Autodesk Inventor part; units mm, degrees
ref_plane "YZ Plane" through (0, 0, 0) normal (1, 0, 0) x (0, 1, 0)
ref_plane "XZ Plane" through (0, 0, 0) normal (0, 1, 0) x (-1, 0, 0)
ref_plane "XY Plane" through (0, 0, 0) normal (0, 0, 1) x (1, 0, 0)
sketch "Sketch1" plane through (0, 0, 0) normal (0, 1, 0) x (-1, 0, 0)
  line L0 (75, 0) -> (75, -100)
  line L1 (75, -100) -> (-75, -100)
  line L2 (-75, -100) -> (-75, 100)
  line L3 (-75, 100) -> (75, 100)
  line L4 (75, 100) -> (75, 0)
  line L5 (75, 100) -> (75, 70)
  line L6 (75, -100) -> (75, -70)
  line L7 (-75, -100) -> (-75, -70)
  line L8 (-75, 100) -> (-75, 70)
  line L9 (75, 70) -> (75, 50)
  line L10 (-75, 70) -> (-75, 50)
  line L11 (-75, -70) -> (-75, -50)
  line L12 (75, -70) -> (75, -50)
  line L13 (75, -70) -> (72.5, -70)
  line L14 (72.5, -70) -> (72.5, -50)
  line L15 (72.5, -50) -> (75, -50)
  line L16 (-75, -70) -> (-72.5, -70)
  line L17 (-72.5, -70) -> (-72.5, -50)
  line L18 (-72.5, -50) -> (-75, -50)
  line L19 (75, 70) -> (72.5, 70)
  line L20 (72.5, 70) -> (72.5, 50)
  line L21 (72.5, 50) -> (75, 50)
  line L22 (-75, 70) -> (-72.5, 70)
  line L23 (-72.5, 70) -> (-72.5, 50)
  line L24 (-72.5, 50) -> (-75, 50)
  line L25 (-75, -100) -> (-75, -97)
  line L26 (-75, -100) -> (-72, -100)
  circle A0 centre (-69.4679, -94.4422) radius 3
  circle A1 centre (69.3699, -94.4422) radius 3
  circle A2 centre (69.3699, 94.4217) radius 3
  circle A3 centre (-69.4679, 94.4217) radius 3
  line L27 (75, -50) -> (75, -35)
  line L28 (75, 50) -> (75, 35)
  line L29 (75, -35) -> (75, -25)
  line L30 (75, 35) -> (75, 25)
  line L31 (75, -25) -> (75, -21)
  line L32 (75, -21) -> (75, -17)
  line L33 (75, -17) -> (75, -13)
  line L34 (75, -13) -> (75, -9)
  line L35 (75, -9) -> (75, -5)
  line L36 (75, -5) -> (75, -1)
  line L37 (75, -1) -> (75, 3)
  line L38 (75, 3) -> (75, 7)
  line L39 (75, 7) -> (75, 11)
  line L40 (75, 11) -> (75, 15)
  line L41 (75, 15) -> (75, 19)
  line L42 (75, 19) -> (75, 23)
  circle A4 centre (60, 30) radius 5
  circle A5 centre (-60, 30) radius 5
  circle A6 centre (0, 30) radius 5
  line L43 (0, -35) -> (0, -30)
  circle A7 centre (0, -30) radius 5
  circle A8 centre (-60, -30) radius 5
  circle A9 centre (60, -30) radius 5
  circle A10 centre (0, -15) radius 2
  circle A11 centre (20, -15) radius 2
  circle A12 centre (44, -15) radius 2
  circle A13 centre (-21, -15) radius 2
  circle A14 centre (-43, -15) radius 2
  circle A15 centre (44, -7) radius 2
  circle A16 centre (20, -7) radius 2
  circle A17 centre (0, -7) radius 2
  circle A18 centre (-21, -7) radius 2
  circle A19 centre (-43, -7) radius 2
  circle A20 centre (44, 1) radius 2
  circle A21 centre (20, 1) radius 2
  circle A22 centre (0, 1) radius 2
  circle A23 centre (-21, 1) radius 2
  circle A24 centre (-43, 1) radius 2
  circle A25 centre (44, 9) radius 2
  circle A26 centre (20, 9) radius 2
  circle A27 centre (0, 9) radius 2
  circle A28 centre (-21, 9) radius 2
  circle A29 centre (-43, 9) radius 2
  circle A30 centre (44, 17) radius 2
  circle A31 centre (20, 17) radius 2
  circle A32 centre (0, 17) radius 2
  circle A33 centre (-21, 17) radius 2
  circle A34 centre (-43, 17) radius 2
  point P0 (0, 0)
  dimension "d3" = 150
  dimension "d4" = 200
  dimension "d6" = 30
  dimension "d7" = 30
  dimension "d8" = 30
  dimension "d9" = 30
  dimension "d10" = 20
  dimension "d11" = 20
  dimension "d12" = 20
  dimension "d13" = 20
  dimension "d14" = 2.5
  dimension "d15" = 2.5
  dimension "d16" = 2.5
  dimension "d17" = 2.5
  dimension "d20" = 6
  dimension "d23" = 6
  dimension "d26" = 6
  dimension "d28" = 6
  dimension "d30" = 15
  dimension "d31" = 15
  dimension "d32" = 10
  dimension "d33" = 10
  dimension "d34" = 4
  dimension "d35" = 4
  dimension "d47" = 10
  dimension "d49" = 10
  dimension "d50" = 10
  dimension "d51" = 5
  dimension "d52" = 10
  dimension "d55" = 10
  dimension "d56" = 10
  dimension "d58" = 4
  dimension "d59" = 4
  dimension "d60" = 4
  dimension "d61" = 4
  dimension "d62" = 4
  dimension "d63" = 4
  dimension "d64" = 4
  dimension "d65" = 4
  dimension "d66" = 4
  dimension "d67" = 4
  dimension "d68" = 4
  dimension "d69" = 4
  dimension "d70" = 4
  dimension "d71" = 4
  dimension "d72" = 4
  dimension "d73" = 4
  dimension "d74" = 4
  dimension "d75" = 4
  dimension "d76" = 4
  dimension "d77" = 4
  dimension "d78" = 4
  dimension "d79" = 4
  dimension "d80" = 4
  dimension "d81" = 4
  dimension "d82" = 4
extrude "Extrusion1" add sketch "Sketch1" along normal blind 5 contours L0 L15 L14 L13 L1 L2 L16 L17 L18 L24 L23 L22 L3 L4 L19 L20 L21
extrude "Extrusion2" add sketch "Sketch1" along normal blind 30 contours L2 L18 L17 L16
extrude "Extrusion3" add sketch "Sketch1" along normal blind 30 contours L0 L13 L14 L15
extrude "Extrusion4" add sketch "Sketch1" along normal blind 30 contours L21 L20 L19 L4
extrude "Extrusion5" add sketch "Sketch1" along normal blind 30 contours L22 L23 L24 L2
sketch "Sketch2" plane through (0, 5, 0) normal (0, 1, 0) x (1, 0, 0)
  point P0 (0, 0)
sketch "Sketch3" plane through (0, 5, 0) normal (0, 1, 0) x (1, 0, 0)
  point P0 (0, 0)
  point P1 (-75, 100)
sketch "Sketch4" plane through (0, 5, 0) normal (0, 1, 0) x (1, 0, 0)
  line L0 (75, 50) -> (70, 50)
  line L1 (70, 50) -> (70, 70)
  line L2 (70, 70) -> (72.5, 70)
  line L3 (72.5, -50) -> (70, -50)
  line L4 (70, -50) -> (70, -70)
  line L5 (70, -70) -> (72.5, -70)
  line L6 (72.5, -70) -> (72.5, -50)
  line L7 (-75, -50) -> (-70, -50)
  line L8 (-70, -50) -> (-70, -70)
  line L9 (-70, -70) -> (-72.5, -70)
  line L10 (-75, 70) -> (-70, 70)
  line L11 (-70, 70) -> (-70, 50)
  line L12 (-70, 50) -> (-72.5, 50)
  line L13 (-72.5, 50) -> (-72.5, 70)
  line L14 (-72.5, -70) -> (-72.5, -50)
  line L15 (72.5, -50) -> (72.5, -70)
  line L16 (72.5, 70) -> (72.5, 50)
  point P0 (0, 0)
  dimension "d93" = 5
  dimension "d95" = 5
extrude "Extrusion6" add sketch "Sketch4" along normal blind 25 contours L10 L11 L12 L13
extrude "Extrusion7" add sketch "Sketch4" along normal blind 25 contours L7 L8 L9 L14
extrude "Extrusion8" add sketch "Sketch4" along normal blind 25 contours L0 L1 L2 L16
extrude "Extrusion9" add sketch "Sketch4" along normal blind 25 contours L6 L5 L4 L3
sketch "Sketch5" plane through (-70, 5, -50) normal (1, 0, 0) x (0, 0, -1)
  point P0 (-50, -5)
sketch "Sketch6" plane through (0, 5, 0) normal (0, 1, 0) x (1, 0, 0)
  point P0 (0, 0)
properties part number "Base"
Geometry check sheet. Reference: the model listing, model coordinates, mm. A direction names the side the tool comes from. Give positions to 0.01 mm unless a question says otherwise; leave off trailing zeros. Write each loop counter-clockwise with the first axis right and the second up, starting at its lowest first coordinate (ties: lowest second). Pieces come first, ordered by that corner, then holes. Notation, with made-up numbers: M 7,30 L 54,30 A17 cw 54,34 Z; hole C 18.25,32.25 d2. An arc over 180 degrees is marked long. One line per question, with ' | ' between items.
1. Cross-section at B-B (y = 7.5). Enter the section's corners in (x, z), plus the area to 3 significant figures.
Ans:
outline: M -75,-70 L -70,-70 L -70,-50 L -75,-50 Z; M -75,50 L -70,50 L -70,70 L -75,70 Z; M 70,-70 L 75,-70 L 75,-50 L 70,-50 Z; M 70,50 L 75,50 L 75,70 L 70,70 Z | area: 400 mm2
2. Cross-section at C-C (z = -64). Enter the section's corners in (x, y), plus the area to 3 significant figures.
Ans:
outline: M -75,0 L 75,0 L 75,30 L 70,30 L 70,5 L -70,5 L -70,30 L -75,30 Z | area: 1,000 mm2
3. Cross-section at A-A (x = -60). Enter the section's corners in (y, z), plus the area to 3 significant figures.
Ans:
outline: M 0,-100 L 5,-100 L 5,-35 L 0,-35 Z; M 0,-25 L 5,-25 L 5,25 L 0,25 Z; M 0,35 L 5,35 L 5,100 L 0,100 Z | area: 900 mm2
4. Scan lines: line 1 along Z through (x, y) = (-44, 3.6); line 2 along Z through (x, y) = (3, 3); line 3 along X through (y, z) = (24, 54). Record each from-to range of solid material in increasing order. Write a range as from..to.
Ans:
line 1: -100..-17, -13..-9, -5..-1, 3..7, 11..15, 19..100 | line 2: -100..-34, -26..26, 34..100 | line 3: -75..-70, 70..75
5. Gauge pin test, flat ends, axial feed: pin 1 (4.5 mm diameter, centred on x = -20, z = 1, fed in from -Y); pin 2 (4 mm diameter, centred on x = -72, y = 12.5, fed in from -Z); pin 3 (11.5 mm diameter, centred on x = 0, z = 30, fed in from +Y); pin 4 (1.5 mm diameter, centred on x = -73, y = 23, fed in from +Z). Record the tip position at first contact, or that the pin passes through.
Ans:
pin 1: y = 0 | pin 2: z = -70 | pin 3: y = 5 | pin 4: z = 70
6. Set-up check for faces 3 (the face through (-70, 17, 60)), 4 (the face through (72, 17, 70)), 5 (the face through (-73, 17, -70)): record each of +Z, -Z, +X, -X, +Y, -Y from which the full face is reachable in a straight line by a thin tool's end or side.
Ans:
face 3: +Z, -Z, +Y | face 4: +Z, +X, -X, +Y | face 5: -Z, +X, -X, +Y
7. Cross-section at D-D (x = 51). Enter the section's corners in (y, z).
Ans:
outline: M 0,-100 L 5,-100 L 5,100 L 0,100 Z
8. Mould release check, pull along X, two halves, no side actions. Record for faces 1 (the face through (-73, 30, -60)), 2 (the face through (0, 2, -9)): released by +X, released by -X, zero draft, split by the parting line, or undercut.
Ans:
face 1: zero draft | face 2: undercut
